```python
from build123d import *

# Parameters (mm, degrees)
SKETCH_1_W      = 20
SKETCH_1_H      = 80
SKETCH_1_R      = 1
EXTRUDE_1_DEPTH = 1.7
SKETCH_3_W      = 5.4
SKETCH_3_H      = 11.2
EXTRUDE_2_DEPTH = 2


with BuildPart() as part:
    # 草图1 → 凸台-拉伸1 (new body)
    with BuildSketch(Plane(origin=(0, 0, 0), x_dir=(1, 0, 0), z_dir=(0, 1, 0))):
        Rectangle(SKETCH_1_W, SKETCH_1_H)
        with Locations(Location((2, 16, 0), (0, 0, 270))):
            Circle(SKETCH_1_R, mode=Mode.SUBTRACT)
        with Locations(Location((2, -16, 0), (0, 0, 270))):
            Circle(SKETCH_1_R, mode=Mode.SUBTRACT)
        with Locations(Location((-7, 37, 0), (0, 0, 270))):
            Circle(SKETCH_1_R, mode=Mode.SUBTRACT)
        with Locations(Location((-7, -37, 0), (0, 0, 270))):
            Circle(SKETCH_1_R, mode=Mode.SUBTRACT)
    extrude(amount=EXTRUDE_1_DEPTH)

    # 草图3 → 凸台-拉伸2 (add)
    with BuildSketch(Plane.XZ):
        with Locations((-7.3, 0)):
            Rectangle(SKETCH_3_W, SKETCH_3_H)
    extrude(amount=EXTRUDE_2_DEPTH)


solid = part.part
```
Source: CAD feature listing. Evaluate the final solid. Frame: model axes, mm. A direction names the side the tool comes from. Round coordinates to 2 decimals unless told otherwise and drop trailing zeros. Loops run counter-clockwise (first coordinate to the right, second up) from the corner with the lowest first, then second, coordinate; pieces in that order, holes last.
1. Section query D-D on x = 7.5. Output: boundary loops of the cut face in (y, z).
2. Mould query, pull axis Z, two halves, no side actions, for faces 1 (the cylindrical face through (-7, 1, -36)), 2 (the flat face through (0, 0, -1)), 3 (the cylindrical face through (2, 1, 17)), 4 (the flat face through (-7, -1, 5.6)). Classes: released by +Z, released by -Z, zero draft, split by the parting line, or undercut.
3. Ray query, L1, parallel to X at y = 0.8, z = -16; L2, parallel to Y at x = 7.75, z = -16.5; L3, parallel to X at y = -1.45, z = -2. Return the intervals inside material, ascending.
4. Section query C-C on y = -0.65. Output: boundary loops of the cut face in (x, z), and give its area (3 significant figures).
5. Contact query for flat-ended pins moving along their axis: pin 1 (3 mm diameter, centred on x = 2, z = 16, fed in from -Y); pin 2 (1.6 mm diameter, centred on x = -7.5, y = -1, fed in from +Z); pin 3 (0.6 mm diameter, centred on x = -8, y = -0.5, fed in from -Z). Output: stop coordinate, or through.
6. Section query A-A on x = 2. Output: boundary loops of the cut face in (y, z).
7. Section query B-B on z = 16. Output: boundary loops of the cut face in (x, y).
8. Access query for faces 5 (the flat face through (-7, -1, -5.6)), 6 (the cylindrical face through (-7, 1, 38)), 7 (the flat face through (-4.6, -1, 0)). Directions: +Z, -Z, +X, -X, +Y, -Y. A direction counts if a zero-diameter tool reaches every point of the face in a straight line with its end or side. Return the directions, or none.
Answers below:
1. outline: (0, -40) - (1.7, -40) - (1.7, 40) - (0, 40) - close
2. face 1: undercut
2. face 2: zero draft
2. face 3: undercut
2. face 4: released by +Z
3. L1: x = -10 to 1, 3 to 10
3. L2: y = 0 to 1.7
3. L3: x = -10 to -4.6
4. outline: (-10, -5.6) - (-4.6, -5.6) - (-4.6, 5.6) - (-10, 5.6) - close
4. area: 60.5 mm2
5. pin 1: stops at y = 0
5. pin 2: stops at z = 5.6
5. pin 3: stops at z = -5.6
6. outline: (0, -40) - (1.7, -40) - (1.7, -17) - (0, -17) - close; (0, -15) - (1.7, -15) - (1.7, 15) - (0, 15) - close; (0, 17) - (1.7, 17) - (1.7, 40) - (0, 40) - close
7. outline: (-10, 0) - (1, 0) - (1, 1.7) - (-10, 1.7) - close; (3, 0) - (10, 0) - (10, 1.7) - (3, 1.7) - close
8. face 5: -Z, +X, -X, -Y
8. face 6: +Y, -Y
8. face 7: +Z, -Z, +X, -Y
